CAD build for the part. Positions are in the model's coordinates, mm. Face numbers are marked on the shaded views. Coordinates: 2 decimals unless noted, no trailing zeros. Loops run counter-clockwise (first coordinate to the right, second up) from the corner with the lowest first, then second, coordinate; pieces in that order, holes last.
1) Saw through at D-D, the plane y = -53.5. Write the cut outline in (x, z).
2) Pin check, flat tips, straight feed: pin 1 Ø1.2 at (y, z) = (47.5, 1.5) entering from -X; pin 2 Ø1 at (x, z) = (-56, 2) entering from +Y; pin 3 Ø1.3 at (x, z) = (-81, 2) entering from +Y. Stop position of each tip, or through.
3) Wall check: line 1 along Y through (x, z) = (-76.5, 5.05); line 2 along X through (y, z) = (64.5, 5.7); line 3 along X through (y, z) = (49.5, 1). Give the ranges that are in metal, low to high.
4) Saw through at C-C, the plane x = -40. Write the cut outline in (y, z).
5) Saw through at B-B, the plane y = -11. Write the cut outline in (x, z).
6) Two-plate mould, pull along Y, no slides. Class the marked faces 1 and 2: +Y half, -Y half, draft (parallel to the pull), parting line (faces both ways), or undercut.
7) Saw through at A-A, the plane z = 2. Write the cut outline in (x, y), and give its area (3 significant figures).
```python
from build123d import *

# Parameters (mm, degrees)
COVER_START                                = 4
COVER_3_2_FOUR_SCREW_CLEARANCES_D3_4_P_R   = 1.7
COVER_3_2_FOUR_SCREW_CLEARANCES_D3_4_DEPTH = 3.2
LOCATING_LIPS_0_45_WALL_CLEARANCE_PROF_W   = 130
LOCATING_LIPS_0_45_WALL_CLEARANCE_PROF_H   = 1.6
LOCATING_LIPS_0_45_WALL_CLEARANCE_PROF_W_2 = 1.6
LOCATING_LIPS_0_45_WALL_CLEARANCE_PROF_H_2 = 70
LOCATING_LIPS_0_45_WALL_CLEARANCE_PROF_H_3 = 12
LOCATING_LIPS_0_45_WALL_CLEARANCE_PROF_H_4 = 73
LOCATING_LIPS_0_45_WALL_CLEARANCE_PROF_H_5 = 15
LOCATING_LIPS_0_45_WALL_CLEARANCE_DEPTH    = 4


with BuildPart() as part:
    # Cover 3.2 - four screw clearances D3.4 profile → Cover 3.2 - four screw clearances D3.4 (new body)
    with BuildSketch(Plane.XY.offset(COVER_START)):
        Polygon((-77, -73), (77, -73), (85, -65), (85, 65), (77, 73), (-77, 73), (-85, 65), (-85, -65), align=None)
        with Locations((-76.5, -64.5)):
            Circle(COVER_3_2_FOUR_SCREW_CLEARANCES_D3_4_P_R, mode=Mode.SUBTRACT)
        with Locations((-76.5, 64.5)):
            Circle(COVER_3_2_FOUR_SCREW_CLEARANCES_D3_4_P_R, mode=Mode.SUBTRACT)
        with Locations((76.5, -64.5)):
            Circle(COVER_3_2_FOUR_SCREW_CLEARANCES_D3_4_P_R, mode=Mode.SUBTRACT)
        with Locations((76.5, 64.5)):
            Circle(COVER_3_2_FOUR_SCREW_CLEARANCES_D3_4_P_R, mode=Mode.SUBTRACT)
    extrude(amount=COVER_3_2_FOUR_SCREW_CLEARANCES_D3_4_DEPTH)

    # Locating lips - 0.45 wall clearance profile → Locating lips - 0.45 wall clearance (add)
    with BuildSketch(Plane.XY):
        with Locations((0, -68.95)):
            Rectangle(LOCATING_LIPS_0_45_WALL_CLEARANCE_PROF_W, LOCATING_LIPS_0_45_WALL_CLEARANCE_PROF_H)
        with Locations((0, 68.95)):
            Rectangle(LOCATING_LIPS_0_45_WALL_CLEARANCE_PROF_W, LOCATING_LIPS_0_45_WALL_CLEARANCE_PROF_H)
        with Locations((-80.95, -16)):
            Rectangle(LOCATING_LIPS_0_45_WALL_CLEARANCE_PROF_W_2, LOCATING_LIPS_0_45_WALL_CLEARANCE_PROF_H_2)
        with Locations((-80.95, 45)):
            Rectangle(LOCATING_LIPS_0_45_WALL_CLEARANCE_PROF_W_2, LOCATING_LIPS_0_45_WALL_CLEARANCE_PROF_H_3)
        with Locations((80.95, -14.5)):
            Rectangle(LOCATING_LIPS_0_45_WALL_CLEARANCE_PROF_W_2, LOCATING_LIPS_0_45_WALL_CLEARANCE_PROF_H_4)
        with Locations((80.95, 43.5)):
            Rectangle(LOCATING_LIPS_0_45_WALL_CLEARANCE_PROF_W_2, LOCATING_LIPS_0_45_WALL_CLEARANCE_PROF_H_5)
    extrude(amount=LOCATING_LIPS_0_45_WALL_CLEARANCE_DEPTH)


solid = part.part
```
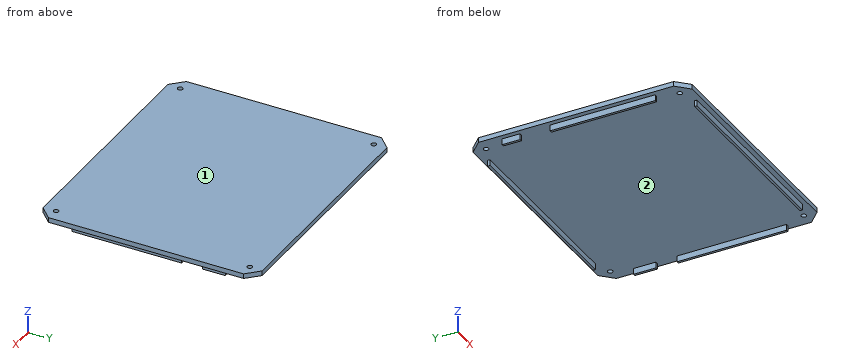
Data:
1. outline: (-85, 4) - (85, 4) - (85, 7.2) - (-85, 7.2) - close
2. pin 1: stops at x = -81.75
2. pin 2: stops at y = 69.75
2. pin 3: stops at y = 51
3. line 1: y = -73 to -66.2, -62.8 to 62.8, 66.2 to 73
3. line 2: x = -85 to -78.2, -74.8 to 74.8, 78.2 to 85
3. line 3: x = -81.75 to -80.15, 80.15 to 81.75
4. outline: (-73, 4) - (-69.75, 4) - (-69.75, 0) - (-68.15, 0) - (-68.15, 4) - (68.15, 4) - (68.15, 0) - (69.75, 0) - (69.75, 4) - (73, 4) - (73, 7.2) - (-73, 7.2) - close
5. outline: (-85, 4) - (-81.75, 4) - (-81.75, 0) - (-80.15, 0) - (-80.15, 4) - (80.15, 4) - (80.15, 0) - (81.75, 0) - (81.75, 4) - (85, 4) - (85, 7.2) - (-85, 7.2) - close
6. face 1: draft
6. face 2: undercut
7. outline: (-81.75, -51) - (-80.15, -51) - (-80.15, 19) - (-81.75, 19) - close; (-81.75, 39) - (-80.15, 39) - (-80.15, 51) - (-81.75, 51) - close; (-65, -69.75) - (65, -69.75) - (65, -68.15) - (-65, -68.15) - close; (-65, 68.15) - (65, 68.15) - (65, 69.75) - (-65, 69.75) - close; (80.15, -51) - (81.75, -51) - (81.75, 22) - (80.15, 22) - close; (80.15, 36) - (81.75, 36) - (81.75, 51) - (80.15, 51) - close
7. area: 688 mm2
